For this review, take the finished solid that the model builds, in its own axes (mm). Give positions to 0.01 mm unless a question says otherwise; leave off trailing zeros. Order: outer loops, then holes, each group sorted by start corner. A loop starts at its lowest first (then second) coordinate and runs counter-clockwise, first axis right, second up. Notation, with made-up numbers: (13.5, 36.25) -> (36.5, 36.25) arc R22 ccw to (36.5, 65.25) -> close; hole circle Ø11 at (46.5, 2.5). An arc over 180 degrees is marked (long way). Return JSON: item names as keys, results as strings. Group by question number.
1) Add section B-B (x = -1.5). Give the boundary of the cut face in (y, z).
2) Insertion check: P1, Ø1.6, axis at y = 1, z = 0.5, coming from the +X side; P2, Ø1, axis at y = 0, z = -42.5, coming from the -X side; P3, Ø2, axis at x = -12, z = 39.5, coming from the -Y side; P4, Ø1.5, axis at x = 12.5, z = 38.5, coming from the -Y side. Each pin has a flat end and moves straight along its axis. Give the tip position at first contact, or say it passes through.
3) Add section A-A (z = -60). Give the boundary of the cut face in (x, y), then the cut area to 3 significant figures.
4) To check wall thickness, follow line 1 along X through (y, z) = (0.05, -11.5); line 2 along Z through (x, y) = (0, -1.55); line 3 along Y through (x, z) = (-17, -52.5). State the ranges of each line that lie inside material, in increasing order.
5) The part is to be moulded in two halves that separate along X. For faces 1 (the face through (0, 0, -72.5)), 2 (the face through (1, 2, 0)), say which applies: released by +X, released by -X, zero draft, split by the parting line, or undercut.
6) Add section C-C (y = -0.75). Give the boundary of the cut face in (x, z), then the cut area to 3 significant figures.
7) Add section D-D (z = -45). Give the boundary of the cut face in (x, y), then the cut area to 3 significant figures.
from build123d import *

# Parameters (mm, degrees)
SKETCH_4_W      = 37
SKETCH_4_H      = 145
EXTRUDE_1_DEPTH = 2
SKETCH_5_W      = 5.125
SKETCH_5_H      = 2
EXTRUDE_2_DEPTH = 2
SKETCH_7_W      = 20.8
SKETCH_7_H      = 2
SKETCH_7_W_2    = 20.5
EXTRUDE_3_DEPTH = 4
EXTRUDE_START   = -37
SKETCH_7_2_W    = 20.8
SKETCH_7_2_H    = 2
SKETCH_7_2_W_2  = 20.5
EXTRUDE_4_DEPTH = 2
EXTRUDE_START_2 = -2.2
EXTRUDE_5_DEPTH = 142.8


with BuildPart() as part:
    # 草图4 → 凸台-拉伸1 (new body)
    with BuildSketch(Plane(origin=(0, 0, 0), x_dir=(1, 0, 0), z_dir=(0, 1, 0))):
        Rectangle(SKETCH_4_W, SKETCH_4_H)
    extrude(amount=EXTRUDE_1_DEPTH)

    # 草图5 → 凸台-拉伸2 (add)
    with BuildSketch(Plane(origin=(0, 0, -72.5), x_dir=(-1, 0, 0), z_dir=(0, 0, -1))):
        with Locations((-15.9375, 1)):
            Rectangle(SKETCH_5_W, SKETCH_5_H)
        with Locations((-5.3125, 1)):
            Rectangle(SKETCH_5_W, SKETCH_5_H)
        with Locations((5.3125, 1)):
            Rectangle(SKETCH_5_W, SKETCH_5_H)
        with Locations((15.9375, 1)):
            Rectangle(SKETCH_5_W, SKETCH_5_H)
    extrude(amount=EXTRUDE_2_DEPTH)

    # 草图7 → 凸台-拉伸3 (add)
    with BuildSketch(Plane(origin=(18.5, 0, 0), x_dir=(0, 0, -1), z_dir=(1, 0, 0))):
        with Locations((-62.1, 1)):
            Rectangle(SKETCH_7_W, SKETCH_7_H)
        with Locations((-19.983333333, 1)):
            Rectangle(SKETCH_7_W_2, SKETCH_7_H)
        with Locations((21.983333333, 1)):
            Rectangle(SKETCH_7_W_2, SKETCH_7_H)
        with Locations((64.1, 1)):
            Rectangle(SKETCH_7_W, SKETCH_7_H)
    extrude(amount=EXTRUDE_3_DEPTH)

    # 草图7<2> → 凸台-拉伸4 (add)
    with BuildSketch(Plane(origin=(18.5, 0, 0), x_dir=(0, 0, -1), z_dir=(1, 0, 0)).offset(EXTRUDE_START)):
        with Locations((-62.1, 1)):
            Rectangle(SKETCH_7_2_W, SKETCH_7_2_H)
        with Locations((-19.983333333, 1)):
            Rectangle(SKETCH_7_2_W_2, SKETCH_7_2_H)
        with Locations((21.983333333, 1)):
            Rectangle(SKETCH_7_2_W_2, SKETCH_7_2_H)
        with Locations((64.1, 1)):
            Rectangle(SKETCH_7_2_W, SKETCH_7_2_H)
    extrude(amount=-EXTRUDE_4_DEPTH)

    # 草图9 → 凸台-拉伸5 (add)
    with BuildSketch(Plane.XY.offset(72.5).offset(EXTRUDE_START_2)):
        Polygon((-9.8, 0), (-11.6, -1.8), (-9.8, -1.8), (9.8, -1.8), (11.6, -1.8), (9.8, 0), align=None)
    extrude(amount=-EXTRUDE_5_DEPTH)


solid = part.part
Evaluation:
{
 "1": {"outline": "(-1.8, -72.5) -> (2, -72.5) -> (2, 72.5) -> (0, 72.5) -> (0, 70.3) -> (-1.8, 70.3) -> close"},
 "2": {"P1": "x = 18.5", "P2": "x = -18.5", "P3": "y = -1.8", "P4": "y = 0"},
 "3": {"outline": "(-20.5, 0) -> (-9.8, 0) -> (-11.6, -1.8) -> (11.6, -1.8) -> (9.8, 0) -> (22.5, 0) -> (22.5, 2) -> (-20.5, 2) -> close", "area": "125 mm^2"},
 "4": {"line 1": "-18.5 to 18.5", "line 2": "-72.5 to 70.3", "line 3": "0 to 2"},
 "5": {"face 1": "undercut", "face 2": "zero draft"},
 "6": {"outline": "(-10.55, -72.5) -> (10.55, -72.5) -> (10.55, 70.3) -> (-10.55, 70.3) -> close", "area": "3,010 mm^2"},
 "7": {"outline": "(-18.5, 0) -> (-9.8, 0) -> (-11.6, -1.8) -> (11.6, -1.8) -> (9.8, 0) -> (18.5, 0) -> (18.5, 2) -> (-18.5, 2) -> close", "area": "113 mm^2"}
}
